For this review, use the dimensioned drawing (mm, ordinates from the lowest corner) and the shaded views. Give positions to 0.01 mm unless a question says otherwise; leave off trailing zeros. Write each loop counter-clockwise with the first axis right and the second up, starting at its lowest first coordinate (ties: lowest second). Pieces come first, ordered by that corner, then holes. Notation, with made-up numbers: (-39.5, -6.75) -> (16.5, -6.75) arc R13 cw to (16.5, 3.25) -> close; hole circle Ø2 at (23, 34.25). An arc over 180 degrees is marked (long way). Answer as CSV lines item,"result".
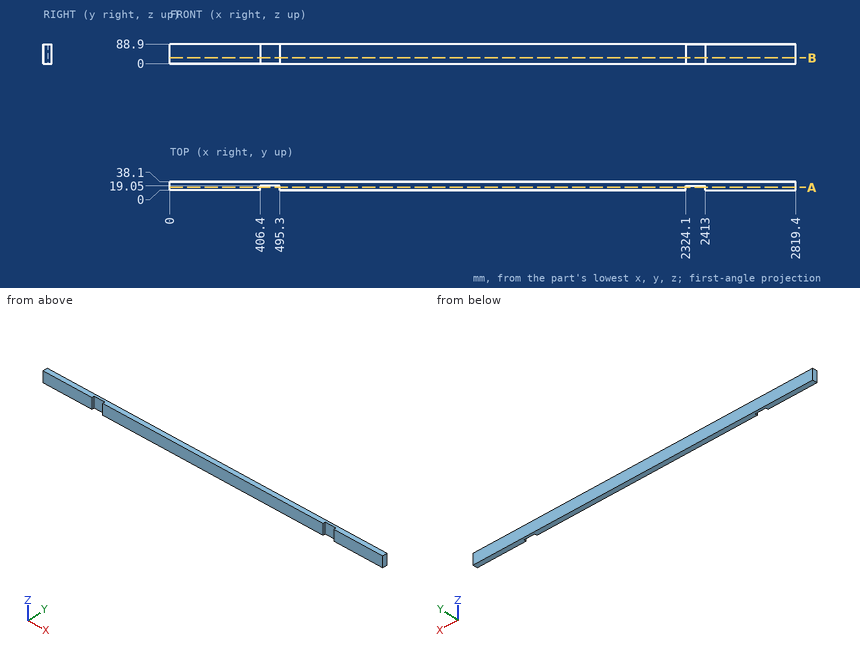
Q1. To check wall thickness, follow probe 1 along X at (y, z) = (2, 26.5); probe 2 along Y at (x, z) = (426.5, 85.5). State the ranges of each line that lie inside material, in increasing order. Write a range as [from, to].
Answer block:
probe 1,"x = [0, 406.4], [495.3, 2324.1], [2413, 2819.4]"
probe 2,"y = [19.05, 38.1]"
Q2. Add section B-B (z = 26). Write out the cut boundary in (x, y), plus the area to 3 significant figures.
Answer block:
outline,"(0, 0) -> (406.4, 0) -> (406.4, 19.05) -> (495.3, 19.05) -> (495.3, 0) -> (2324.1, 0) -> (2324.1, 19.05) -> (2413, 19.05) -> (2413, 0) -> (2819.4, 0) -> (2819.4, 38.1) -> (0, 38.1) -> close"
area,"104,000 mm2"
Q3. Add section A-A (y = 12.5). Write out the cut boundary in (x, z).
Answer block:
outline,"(0, 0) -> (406.4, 0) -> (406.4, 88.9) -> (0, 88.9) -> close; (495.3, 0) -> (2324.1, 0) -> (2324.1, 88.9) -> (495.3, 88.9) -> close; (2413, 0) -> (2819.4, 0) -> (2819.4, 88.9) -> (2413, 88.9) -> close"
